Input: part model. Units: mm. Frame: model coordinates. A direction names the side the tool comes from. Round coordinates to 2 decimals unless told otherwise and drop trailing zeros. Order: outer loops, then holes, each group sorted by start corner. A loop starts at its lowest first (then second) coordinate and runs counter-clockwise, first axis right, second up. Notation, with made-up numbers: (77, 71) -> (113, 71) arc R17 cw to (113, 79) -> close; hole circle Ø8 at (69, -8). An arc over 180 degrees is marked (long way). Use a Markdown table: item, result.
from build123d import *

# Parameters (mm, degrees)
SKETCH1_R           = 87.5
BOSS_EXTRUDE1_DEPTH = 29
SKETCH2_R           = 25
CUT_EXTRUDE1_DEPTH  = 128.096420091
SKETCH3_R           = 9.921747731
CUT_EXTRUDE2_DEPTH  = 20.272624
CIRPATTERN1_START   = 8.727375649
CIRPATTERN1_DEPTH   = 20.272624351


# Read off the part's stored shape, not the designer's step: CirPattern1
with BuildPart() as part:
    # Sketch1 → Boss-Extrude1 (new body)
    with BuildSketch(Plane(origin=(0, 0, 0), x_dir=(1, 0, 0), z_dir=(0, 1, 0))):
        with Locations(Location((0, 0, 0), (0, 0, 90))):
            Circle(SKETCH1_R)
    extrude(amount=BOSS_EXTRUDE1_DEPTH)

    # Sketch2 → Cut-Extrude1 (cut, through all)
    with BuildSketch(Plane(origin=(0, 0, 0), x_dir=(1, 0, 0), z_dir=(0, 1, 0))):
        with Locations(Location((0, 0, 0), (0, 0, 90))):
            Circle(SKETCH2_R)
    extrude(amount=CUT_EXTRUDE1_DEPTH, mode=Mode.SUBTRACT)

    # Sketch3 → Cut-Extrude2 (cut)
    with BuildSketch(Plane(origin=(0, 29, 0), x_dir=(1, 0, 0), z_dir=(0, 1, 0))):
        with Locations((-32.93055591, 0)):
            Circle(SKETCH3_R)
    extrude(amount=-CUT_EXTRUDE2_DEPTH, mode=Mode.SUBTRACT)

    # CirPattern1 outline → CirPattern1 (cut)
    with BuildSketch(Plane(origin=(0, 0, 0), x_dir=(1, 0, 0), z_dir=(0, 1, 0)).offset(CIRPATTERN1_START)):
        with BuildLine():
            ThreePointArc((-7.755597806, -23.766587948), (-12.5, -21.650635095), (-16.704670021, -18.599838696))
            ThreePointArc((-16.704670021, -18.599838696), (-21.426151818, -37.111183564), (-7.755597806, -23.766587948))
        make_face()
        with BuildLine():
            ThreePointArc((-7.755597806, 23.766587947), (-21.426151818, 37.111183564), (-16.704670021, 18.599838696))
            ThreePointArc((-16.704670021, 18.599838696), (-12.5, 21.650635095), (-7.755597806, 23.766587947))
        make_face()
        with BuildLine():
            ThreePointArc((16.704670021, -18.599838696), (12.5, -21.650635095), (7.755597806, -23.766587948))
            ThreePointArc((7.755597806, -23.766587948), (21.426151818, -37.111183564), (16.704670021, -18.599838696))
        make_face()
        with BuildLine():
            ThreePointArc((16.704670021, 18.599838696), (21.426151818, 37.111183564), (7.755597806, 23.766587947))
            ThreePointArc((7.755597806, 23.766587947), (12.5, 21.650635095), (16.704670021, 18.599838696))
        make_face()
        with BuildLine():
            ThreePointArc((24.460267827, 5.166749252), (25, 0), (24.460267827, -5.166749252))
            ThreePointArc((24.460267827, -5.166749252), (42.85230364, 0), (24.460267827, 5.166749252))
        make_face()
    extrude(amount=CIRPATTERN1_DEPTH, mode=Mode.SUBTRACT)


solid = part.part
1) Set-up query: faces 4 (the cylindrical face through (22.2, 14.3, -11.5)), 5 (the flat face through (16, 8.727, -29)). Return all of +Z, -Z, +X, -X, +Y, -Y with unobstructed straight access to the full face (end or side cutting, diameter ignored); none if empty.
Results found:
| item | result |
|---|---|
| face 4 | +Y, -Y |
| face 5 | +Y |
2) Pin query (flat end, axial travel): pin 1 Ø9 at (x, z) = (34.5, 4.5) entering from +Y; pin 2 Ø5 at (y, z) = (25.5, 53.5) entering from +X; pin 3 Ø12 at (y, z) = (21, -27) entering from +X. Return the tip coordinate at first contact, or that it passes through.
Results found:
| item | result |
|---|---|
| pin 1 | stops at y = 8.73 |
| pin 2 | stops at x = 71.1 |
| pin 3 | stops at x = 84.94 |
3) Cut plane C-C on y = 20.25. Return loops of the section in (x, z).
Results found:
| item | result |
|---|---|
| outline | circle Ø175 at (0, 0); hole (-24.46, -5.17) arc R25 ccw to (-16.7, -18.6) arc R9.92 ccw (long way) to (-7.76, -23.77) arc R25 ccw to (7.76, -23.77) arc R9.92 ccw (long way) to (16.7, -18.6) arc R25 ccw to (24.46, -5.17) arc R9.92 ccw (long way) to (24.46, 5.17) arc R25 ccw to (16.7, 18.6) arc R9.92 ccw (long way) to (7.76, 23.77) arc R25 ccw to (-7.76, 23.77) arc R9.92 ccw (long way) to (-16.7, 18.6) arc R25 ccw to (-24.46, 5.17) arc R9.92 ccw (long way) to start |
4) Cut plane A-A on z = 0. Return loops of the section in (x, y).
Results found:
| item | result |
|---|---|
| outline | (-87.5, 0) -> (-25, 0) -> (-25, 8.73) -> (-42.85, 8.73) -> (-42.85, 29) -> (-87.5, 29) -> close; (25, 0) -> (87.5, 0) -> (87.5, 29) -> (42.85, 29) -> (42.85, 8.73) -> (25, 8.73) -> close |
5) Pull-direction query (X, two-part tool) for faces 1 (the flat face through (34, 8.727, 0)), 2 (the cylindrical face through (-86.755, 14.297, 11.391)), 3 (the flat face through (18, 29, -18)); classes: +X half, -X half, draft (parallel to the pull), parting line (faces both ways), or undercut.
Results found:
| item | result |
|---|---|
| face 1 | undercut |
| face 2 | parting line |
| face 3 | draft |
6) Line query: L1, parallel to X at y = 24.25, z = 0; L2, parallel to Z at x = -1, y = 3.5; L3, parallel to Z at x = -7.5, y = 23.75. Output: solid intervals per line, ascending. Write a range as [from, to].
Results found:
| item | result |
|---|---|
| L1 | x = [-87.5, -42.85], [42.85, 87.5] |
| L2 | z = [-87.49, -24.98], [24.98, 87.49] |
| L3 | z = [-87.18, -32.77], [-24.27, -23.85], [23.85, 24.27], [32.77, 87.18] |
7) Cut plane B-B on x = 0. Return loops of the section in (y, z).
Results found:
| item | result |
|---|---|
| outline | (0, -87.5) -> (29, -87.5) -> (29, -25) -> (0, -25) -> close; (0, 25) -> (29, 25) -> (29, 87.5) -> (0, 87.5) -> close |
8) Cut plane D-D on x = -20. Return loops of the section in (y, z).
Results found:
| item | result |
|---|---|
| outline | (0, -85.18) -> (29, -85.18) -> (29, -37.79) -> (8.73, -37.79) -> (8.73, -19.25) -> (29, -19.25) -> (29, -15) -> (0, -15) -> close; (0, 15) -> (29, 15) -> (29, 19.25) -> (8.73, 19.25) -> (8.73, 37.79) -> (29, 37.79) -> (29, 85.18) -> (0, 85.18) -> close |
